from build123d import *

# Parameters (mm, degrees)
BOSS_EXTRUDE1_DEPTH = 10
BOSS_EXTRUDE2_DEPTH = 5
CUT_EXTRUDE1_START  = 30
CUT_EXTRUDE1_DEPTH  = 25
CUT_EXTRUDE2_REACH  = 55.151
SKETCH4_R           = 1.4


with BuildPart() as part:
    # Sketch1 → Boss-Extrude1 (new body)
    with BuildSketch(Plane(origin=(0, 0, 0), x_dir=(1, 0, 0), z_dir=(0, 1, 0))):
        Polygon((-5.1, 15), (-5.1, 8), (5.1, 8), (5.1, 15), (10, 15), (10, -15), (-10, -15), (-10, 15), align=None)
    extrude(amount=BOSS_EXTRUDE1_DEPTH)

    # Sketch2 → Boss-Extrude2 (add, symmetric)
    with BuildSketch(Plane(origin=(0, 0, 0), x_dir=(0, 0, -1), z_dir=(1, 0, 0))):
        Polygon((-15, 10), (8, 50), (8, 10), align=None)
    extrude(amount=BOSS_EXTRUDE2_DEPTH, both=True)

    # Sketch3 → Cut-Extrude1 (cut)
    with BuildSketch(Plane(origin=(0, 0, 0), x_dir=(1, 0, 0), z_dir=(0, 1, 0)).offset(CUT_EXTRUDE1_START)):
        Polygon((3.117691454, -7), (1.558845727, -4.3), (-1.558845727, -4.3), (-3.117691454, -7), (-1.558845727, -9.7), (1.558845727, -9.7), align=None)
    extrude(amount=-CUT_EXTRUDE1_DEPTH, mode=Mode.SUBTRACT)

    # Sketch4 → Cut-Extrude2 (cut, up to next)
    with BuildSketch(Plane(origin=(0, 0, 0), x_dir=(1, 0, 0), z_dir=(0, 1, 0)), mode=Mode.PRIVATE) as cut_extrude2_sk1:
        with Locations(Location((0, -7, 0), (0, 0, 270))):
            Circle(SKETCH4_R)
    cut_extrude2_tool1 = extrude(cut_extrude2_sk1.sketch, amount=CUT_EXTRUDE2_REACH, mode=Mode.PRIVATE) & part.part
    add(cut_extrude2_tool1.solids().sort_by_distance((0, 0, 7))[0], mode=Mode.SUBTRACT)


solid = part.part
Here's how the part is built. I have some questions about the finished solid (model axes, mm). A direction names the side the tool comes from. Give positions to 0.01 mm unless a question says otherwise; leave off trailing zeros. Order: outer loops, then holes, each group sorted by start corner. A loop starts at its lowest first (then second) coordinate and runs counter-clockwise, first axis right, second up. Notation, with made-up numbers: M -25,-33.75 L 27,-33.75 A20 ccw 27,-1.75 Z; hole C 55,88 d9. An arc over 180 degrees is marked long. Answer as a JSON object with one key per item and string values. Group by question number.
1) We'd pull the mould along X, two halves only. Please class faces 1 (the flat face through (0, 25, -8)), 2 (the flat face through (-2.327, 16.97, 5.631)), 3 (the flat face through (8, 10, 0)), 4 (the flat face through (10, 5, 0)): pulls with the +X half, pulls with the -X half, needs draft (parallel to the pull), parting line crosses it, or undercut.
2) On a 3-axis mill with a long thin cutter (end or side, diameter ignored), from which of +Z, -Z, +X, -X, +Y, -Y can I reach the whole of each face in a straight line? I mean faces 5 (the flat face through (0.07, 29.72, 3.66)), 6 (the flat face through (0, 17, 4.3)), 7 (the flat face through (5, 21, -2)), 8 (the flat face through (5.1, 5, -11)), 9 (the flat face through (-5, 21, -2)). Say none if no direction works.
3) Suppose I cut it at A-A, the plane x = 0. Write out the boundary of the cut face in (y, z), plus the area to 3 significant figures.
4) Please list where these lines run through material, in increasing order: L1, parallel to X at y = 3.6, z = 7; L2, parallel to Z at x = 0, y = 3; L3, parallel to X at y = 9.5, z = -10.5. Write a range as [from, to].
5) I'm going to push flat-ended pins straight in: pin 1 Ø6 at (x, z) = (-1, 6.5) entering from +Y; pin 2 Ø1.5 at (x, z) = (-7.5, -2) entering from +Y; pin 3 Ø1.5 at (y, z) = (27, -6.5) entering from +X; pin 4 Ø8 at (x, z) = (-3.5, -8) entering from -Y. Where does each tip first touch, or does it pass through?
6) Suppose I cut it at B-B, the plane z = -11.5. Write out the boundary of the cut face in (x, y), plus the area to 3 significant figures.
7) Suppose I cut it at D-D, the plane x = -4.5. Write out the boundary of the cut face in (y, z).
8) Suppose I cut it at C-C, the plane y = 22.5. Write out the boundary of the cut face in (x, z).
Results found:
{
 "1": {"face 1": "undercut", "face 2": "undercut", "face 3": "needs draft", "face 4": "pulls with the +X half"},
 "2": {"face 5": "+Z, +X, -X, +Y", "face 6": "+Y", "face 7": "+Z, -Z, +X, +Y", "face 8": "-Z, +Y, -Y", "face 9": "+Z, -Z, -X, +Y"},
 "3": {"outline": "M 0,-8 L 50,-8 L 28.61,4.3 L 5,4.3 L 5,5.6 L 0,5.6 Z; M 0,8.4 L 5,8.4 L 5,9.7 L 19.22,9.7 L 10,15 L 0,15 Z", "area": "574 mm²"},
 "4": {"L1": "[-10, -1.4], [1.4, 10]", "L2": "[-8, 5.6], [8.4, 15]", "L3": "[-10, -5.1], [5.1, 10]"},
 "5": {"pin 1": "y = 30", "pin 2": "y = 10", "pin 3": "x = 5", "pin 4": "y = 0"},
 "6": {"outline": "M -10,0 L -5.1,0 L -5.1,10 L -10,10 Z; M 5.1,0 L 10,0 L 10,10 L 5.1,10 Z", "area": "98.0 mm²"},
 "7": {"outline": "M 0,-8 L 50,-8 L 10,15 L 0,15 Z"},
 "8": {"outline": "M -5,-8 L 5,-8 L 5,7.81 L 2.65,7.81 L 3.12,7 L 1.56,4.3 L -1.56,4.3 L -3.12,7 L -2.65,7.81 L -5,7.81 Z"}
}
